Work out the finished part from the listing and answer in its coordinate system (mm). Face numbers are marked on the shaded views. A direction names the side the tool comes from. Coordinates: 2 decimals unless noted, no trailing zeros. Order: outer loops, then holes, each group sorted by start corner. A loop starts at its lowest first (then second) coordinate and runs counter-clockwise, first axis right, second up. Notation, with made-up numbers: M -9.5,20.25 L 10.5,20.25 A28 cw 10.5,51.25 Z; hole C 60,24 d2. An arc over 180 degrees is marked long. Use a Markdown table: item, result. Add a question column.
Autodesk Inventor part; units mm, degrees
ref_plane "YZ Plane" through (0, 0, 0) normal (1, 0, 0) x (0, 1, 0)
ref_plane "XZ Plane" through (0, 0, 0) normal (0, 1, 0) x (-1, 0, 0)
ref_plane "XY Plane" through (0, 0, 0) normal (0, 0, 1) x (1, 0, 0)
sketch "Sketch1" plane through (0, 0, 0) normal (0, 0, 1) x (1, 0, 0)
  line L0 (0, 0) -> (25.4, 0)
  line L1 (25.4, 0) -> (25.4, 25.4)
  line L2 (25.4, 25.4) -> (0, 25.4)
  line L3 (0, 25.4) -> (0, 0)
  dimension "d0" = 25.4
  dimension "d1" = 25.4
extrude "Extrusion1" add sketch "Sketch1" along normal blind 177.8
shell "Shell1" thickness 1.5875 removed faces 2 at (8.4667, 16.9333, 0) at (8.4667, 16.9333, 177.8)
sketch "Sketch2" plane through (0, 25.4, 0) normal (0, 1, 0) x (1, 0, 0)
  line L0 (0, -177.8) -> (25.4, -177.8)
  line L1 (25.4, 0) -> (0, 0)
  line L2 (0, 0) -> (0, -177.8)
  line L3 (0, 0) -> (0, -14.6647)
  line L4 (25.4, 0) -> (0, -14.6647)
  line L5 (0, 0) -> (25.4, 0)
  line L6 (0, -133.8059) -> (0, -177.8)
  line L7 (0, -177.8) -> (25.4, -177.8)
  line L8 (0, -133.8059) -> (25.4, -177.8)
  dimension "d5" = 60
  dimension "d6" = 30
extrude "Extrusion2" cut sketch "Sketch2" against normal through all
properties part number "Frame_FrontAngle" material "Aluminum-6061"
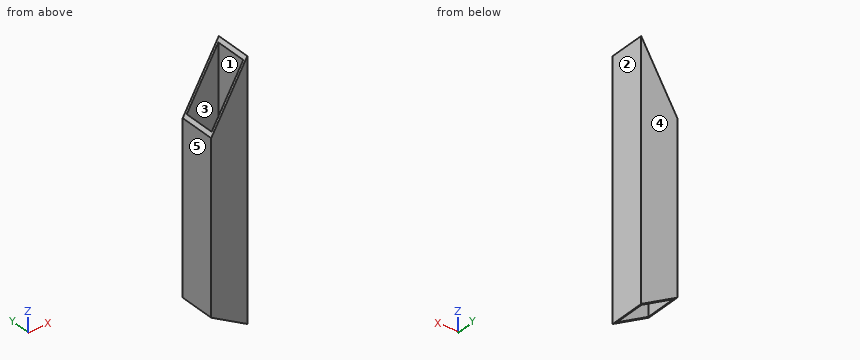
(1) Straight lines are drawn through the part: line 1 (X direction, y = 10.5, z = 51); line 2 (X direction, y = 15, z = 156.5). For each, find the intervals that lie inside material, in ascending order.
(2) A cutting plane is placed at B-B on z = 103. Write down the section's boundary in (x, y).
(3) A cutting plane is placed at D-D on z = 144.5. Write down the section's boundary in (x, y).
(4) A cutting plane is placed at C-C on x = 8. Write down the section's boundary in (y, z), plus the area to 3 significant figures.
(5) Which of the six approach directions +Z, -Z, +X, -X, +Y, -Y give full straight-line access (tool end or side, diameter ignored) to the marked faces 1 and 2?
(6) Given P1, Ø12, axis at y = 16.5, z = 35, coming from the -X side; P2, Ø4, axis at y = 10, z = 137, coming from the -X side, each flat-ended and moving along its own axis, determine where each tip first touches the part or whether it passes through.
(7) The mould has two halves that part along X. Classify the marked faces 3, 4 and 5: pulls with the +X half, pulls with the -X half, needs draft (parallel to the pull), parting line crosses it, or undercut.
(8) A cutting plane is placed at A-A on y = 8. Write down the section's boundary in (x, z).
From the geometry:
| question | item | result |
|---|---|---|
| 1 | line 1 | x = 0 to 1.59, 23.81 to 25.4 |
| 1 | line 2 | x = 23.81 to 25.4 |
| 2 | outline | M 0,0 L 25.4,0 L 25.4,25.4 L 0,25.4 Z; hole M 1.59,1.59 L 23.81,1.59 L 23.81,23.81 L 1.59,23.81 Z |
| 3 | outline | M 6.17,0 L 25.4,0 L 25.4,25.4 L 6.17,25.4 L 6.17,23.81 L 23.81,23.81 L 23.81,1.59 L 6.17,1.59 Z |
| 4 | outline | M 0,10.05 L 1.59,10.05 L 1.59,147.66 L 0,147.66 Z; M 23.81,10.05 L 25.4,10.05 L 25.4,147.66 L 23.81,147.66 Z |
| 4 | area | 437 mm2 |
| 5 | face 1 | +Z, -Z |
| 5 | face 2 | +Z, -Z, +X, +Y, -Y |
| 6 | P1 | stops at x = 0 |
| 6 | P2 | stops at x = 0.69 |
| 7 | face 3 | undercut |
| 7 | face 4 | needs draft |
| 7 | face 5 | pulls with the -X half |
| 8 | outline | M 0,14.66 L 1.59,13.75 L 1.59,136.56 L 0,133.81 Z; M 23.81,0.92 L 25.4,0 L 25.4,177.8 L 23.81,175.05 Z |
